```python
from build123d import *

# Parameters (mm, degrees)
ESBO_O1_R                = 45
RESSALTO_EXTRUS_O1_DEPTH = 50
ESBO_O2_R                = 4.5
CORTE_EXTRUS_O2_DEPTH    = 6
CORTE_EXTRUS_O3_DEPTH    = 7
ESBO_O4_W                = 40
ESBO_O4_H                = 15
CORTE_EXTRUS_O4_DEPTH    = 41
CORTE_EXTRUS_O5_START    = -6
ESBO_O5_R                = 4.5
CORTE_EXTRUS_O5_DEPTH    = 6
CORTE_EXTRUS_O6_START    = -7
CORTE_EXTRUS_O6_DEPTH    = 7
ESBO_O7_W                = 40
ESBO_O7_H                = 15
CORTE_EXTRUS_O7_DEPTH    = 47
CORTE_EXTRUS_O8_REACH    = 72.356
CORTE_EXTRUS_O9_REACH    = 72.356
ESBO_O9_W                = 5.8
ESBO_O9_H                = 3.2
ESBO_O11_W               = 40
ESBO_O11_H               = 15
ESBO_O11_W_2             = 13
ESBO_O11_H_2             = 7
RESSALTO_EXTRUS_O2_DEPTH = 22
ESBO_O12_R               = 1.6
CORTE_EXTRUS_O10_DEPTH   = 10
CORTE_EXTRUS_O11_REACH   = 75.614
ESBO_O13_R               = 4.5


with BuildPart() as part:
    # Esboço1 → Ressalto-extrusão1 (new body)
    with BuildSketch(Plane.XY):
        Circle(ESBO_O1_R)
    extrude(amount=RESSALTO_EXTRUS_O1_DEPTH)

    # Esboço2 → Corte-extrusão2 (cut)
    with BuildSketch(Plane.XY.offset(50)):
        Circle(ESBO_O2_R)
    extrude(amount=-CORTE_EXTRUS_O2_DEPTH, mode=Mode.SUBTRACT)

    # Esboço3 → Corte-extrusão3 (cut)
    with BuildSketch(Plane.XY.offset(44)):
        with BuildLine():
            Line((-6.5, -3.073450829), (-6.5, 7.19))
            Line((-6.5, 7.19), (6.5, 7.19))
            Line((6.5, 7.19), (6.5, -3.073450829))
            ThreePointArc((6.5, -3.073450829), (0, -7.19), (-6.5, -3.073450829))
        make_face()
    extrude(amount=-CORTE_EXTRUS_O3_DEPTH, mode=Mode.SUBTRACT)

    # Esboço4 → Corte-extrusão4 (cut)
    with BuildSketch(Plane.XZ.offset(-7.19)):
        with Locations((0, 37.5)):
            Rectangle(ESBO_O4_W, ESBO_O4_H)
    extrude(amount=-CORTE_EXTRUS_O4_DEPTH, mode=Mode.SUBTRACT)

    # Esboço5 → Corte-extrusão5 (cut)
    with BuildSketch(Plane(origin=(0, 0, 0), x_dir=(-1, 0, 0), z_dir=(0, 0, -1)).offset(CORTE_EXTRUS_O5_START)):
        with Locations(Location((0, 0, 0), (0, 0, 180))):
            Circle(ESBO_O5_R)
    extrude(amount=CORTE_EXTRUS_O5_DEPTH, mode=Mode.SUBTRACT)

    # Esboço6 → Corte-extrusão6 (cut)
    with BuildSketch(Plane(origin=(0, 0, 6), x_dir=(-1, 0, 0), z_dir=(0, 0, -1)).offset(CORTE_EXTRUS_O6_START)):
        with BuildLine():
            Line((-6.5, -3.073450829), (-6.5, 7.19))
            Line((-6.5, 7.19), (6.5, 7.19))
            Line((6.5, 7.19), (6.5, -3.073450829))
            ThreePointArc((6.5, -3.073450829), (0, -7.19), (-6.5, -3.073450829))
        make_face()
    extrude(amount=CORTE_EXTRUS_O6_DEPTH, mode=Mode.SUBTRACT)

    # Esboço7 → Corte-extrusão7 (cut)
    with BuildSketch(Plane.XZ.offset(-7.19)):
        with Locations((0, 12.5)):
            Rectangle(ESBO_O7_W, ESBO_O7_H)
    extrude(amount=-CORTE_EXTRUS_O7_DEPTH, mode=Mode.SUBTRACT)

    # Esboço8 → Corte-extrusão8 (cut, up to next)
    with BuildSketch(Plane.XY.offset(30), mode=Mode.PRIVATE) as corte_extrus_o8_sk1:
        Polygon((-20, 40.311288741), (-20, 47.3700993), (20, 47.3700993), (20, 40.311288741), (20, 37.311288741), (-20, 37.311288741), align=None)
    corte_extrus_o8_tool1 = extrude(corte_extrus_o8_sk1.sketch, amount=-CORTE_EXTRUS_O8_REACH, mode=Mode.PRIVATE) & part.part
    add(corte_extrus_o8_tool1.solids().sort_by_distance((0, 42.340694, 30))[0], mode=Mode.SUBTRACT)

    # Esboço9 → Corte-extrusão9 (cut, up to next)
    with BuildSketch(Plane(origin=(0, 0, 20), x_dir=(-1, 0, 0), z_dir=(0, 0, -1)), mode=Mode.PRIVATE) as corte_extrus_o9_sk1:
        with Locations((-15.1, 32.711288741)):
            Rectangle(ESBO_O9_W, ESBO_O9_H)
    corte_extrus_o9_tool1 = extrude(corte_extrus_o9_sk1.sketch, amount=-CORTE_EXTRUS_O9_REACH, mode=Mode.PRIVATE) & part.part
    # Esboço9 → Corte-extrusão9 (cut, up to next)
    with BuildSketch(Plane(origin=(0, 0, 20), x_dir=(-1, 0, 0), z_dir=(0, 0, -1)), mode=Mode.PRIVATE) as corte_extrus_o9_sk2:
        with Locations((15.1, 32.711288741)):
            Rectangle(ESBO_O9_W, ESBO_O9_H)
    corte_extrus_o9_tool2 = extrude(corte_extrus_o9_sk2.sketch, amount=-CORTE_EXTRUS_O9_REACH, mode=Mode.PRIVATE) & part.part
    add(corte_extrus_o9_tool1.solids().sort_by_distance((15.1, 32.711289, 20))[0], mode=Mode.SUBTRACT)
    add(corte_extrus_o9_tool2.solids().sort_by_distance((-15.1, 32.711289, 20))[0], mode=Mode.SUBTRACT)

    # Esboço11 → Ressalto-extrusão2 (add)
    # profile 1 of 2: a face of its own
    with BuildSketch(Plane(origin=(0, 7.19, 0), x_dir=(1, 0, 0), z_dir=(0, 1, 0))):
        with Locations((0, -12.5)):
            Rectangle(ESBO_O11_W, ESBO_O11_H)
        with Locations((0, -9.5)):
            Rectangle(ESBO_O11_W_2, ESBO_O11_H_2, mode=Mode.SUBTRACT)
    # profile 2 of 2: a face of its own
    with BuildSketch(Plane(origin=(0, 7.19, 0), x_dir=(1, 0, 0), z_dir=(0, 1, 0))):
        with Locations((0, -37.5)):
            Rectangle(ESBO_O11_W, ESBO_O11_H)
        with Locations((0, -40.5)):
            Rectangle(ESBO_O11_W_2, ESBO_O11_H_2, mode=Mode.SUBTRACT)
    extrude(amount=RESSALTO_EXTRUS_O2_DEPTH)

    # Esboço12 → Corte-extrusão10 (cut)
    with BuildSketch(Plane(origin=(0, 37.311288741, 0), x_dir=(1, 0, 0), z_dir=(0, 1, 0))):
        with Locations(Location((-15.1, -25, 0), (0, 0, 270))):
            Circle(ESBO_O12_R)
        with Locations(Location((15.1, -25, 0), (0, 0, 270))):
            Circle(ESBO_O12_R)
    extrude(amount=-CORTE_EXTRUS_O10_DEPTH, mode=Mode.SUBTRACT)

    # Esboço13 → Corte-extrusão11 (cut, up to next)
    with BuildSketch(Plane.XY.offset(37), mode=Mode.PRIVATE) as corte_extrus_o11_sk1:
        Circle(ESBO_O13_R)
    corte_extrus_o11_tool1 = extrude(corte_extrus_o11_sk1.sketch, amount=-CORTE_EXTRUS_O11_REACH, mode=Mode.PRIVATE) & part.part
    add(corte_extrus_o11_tool1.solids().sort_by_distance((0, 0, 37))[0], mode=Mode.SUBTRACT)


solid = part.part
```
Geometry: final body of the model. Coordinates: model frame, mm. A direction names the side the tool comes from. Give positions to 0.01 mm unless a question says otherwise; leave off trailing zeros. Loops run counter-clockwise (first coordinate to the right, second up) from the corner with the lowest first, then second, coordinate; pieces in that order, holes last. Notation, with made-up numbers: (-2.5, 33.5) -> (1.5, 33.5) arc R14 cw to (1.5, 45.5) -> close; hole circle Ø6 at (61, 74.5). An arc over 180 degrees is marked (long way). Use CSV: the item, a comma, the result in double quotes.
(1) Pull-direction query (Y, two-part tool) for faces 4 (the face through (18, 33, 25)), 5 (the face through (0, 33, 20)), 6 (the face through (20.765, -39.923, 24.65)); classes: released by +Y, released by -Y, zero draft, split by the parting line, or undercut.
From the geometry:
face 4,"undercut"
face 5,"zero draft"
face 6,"split by the parting line"
(2) Cut plane C-C (z = 39). Output: boundary loops of the cut face in (x, y).
From the geometry:
outline,"(-20, 29.19) -> (-20, 40.31) arc R45 ccw (long way) to (20, 40.31) -> (20, 29.19) -> (6.5, 29.19) -> (6.5, -3.07) arc R7.19 cw to (-6.5, -3.07) -> (-6.5, 29.19) -> close"
(3) First-contact query: P1, Ø6.5, axis at x = -14, z = 22.5, coming from the +Y side; P2, Ø12, axis at y = -14, z = 30.5, coming from the +X side; P3, Ø8, axis at x = -22.5, z = 11.5, coming from the -Y side; P4, Ø7, axis at x = 0, y = 0, coming from the +Z side. Flat tips, straight axial feed; report the tip coordinate or a pass-through.
From the geometry:
P1,"y = 37.31"
P2,"x = 44.28"
P3,"y = -41.02"
P4,"through"
(4) Access query for faces 1 (the face through (-0.11, -7.19, 9.55)), 2 (the face through (-18, 33, 25)), 3 (the face through (-3.32, -3.04, 3.04)). Directions: +Z, -Z, +X, -X, +Y, -Y. A direction counts if a zero-diameter tool reaches every point of the face in a straight line with its end or side. Return the directions, or none.
From the geometry:
face 1,"+Y"
face 2,"none"
face 3,"+Z, -Z"
(5) Cut plane B-B (y = 0). Output: boundary loops of the cut face in (x, z), plus the area to 3 significant figures.
From the geometry:
outline,"(-45, 0) -> (-4.5, 0) -> (-4.5, 6) -> (-6.5, 6) -> (-6.5, 13) -> (-4.5, 13) -> (-4.5, 37) -> (-6.5, 37) -> (-6.5, 44) -> (-4.5, 44) -> (-4.5, 50) -> (-45, 50) -> close; (4.5, 0) -> (45, 0) -> (45, 50) -> (4.5, 50) -> (4.5, 44) -> (6.5, 44) -> (6.5, 37) -> (4.5, 37) -> (4.5, 13) -> (6.5, 13) -> (6.5, 6) -> (4.5, 6) -> close"
area,"3,990 mm^2"
(6) Cut plane D-D (y = 10). Output: boundary loops of the cut face in (x, z).
From the geometry:
outline,"(-43.87, 0) -> (43.87, 0) -> (43.87, 50) -> (-43.87, 50) -> close; hole (-6.5, 6) -> (6.5, 6) -> (6.5, 13) -> (-6.5, 13) -> close; hole (-6.5, 37) -> (6.5, 37) -> (6.5, 44) -> (-6.5, 44) -> close"
(7) Ray query, line 1 along Z through (x, y) = (15, 35); line 2 along Y through (x, z) = (0, 48.7); line 3 along Z through (x, y) = (1, 14). Return the intervals inside material, ascending. Write a range as [from, to].
From the geometry:
line 1,"[0, 5], [20, 23.4], [26.6, 30], [45, 50]"
line 2,"[-45, -4.5], [4.5, 45]"
line 3,"[0, 6], [13, 37], [44, 50]"
(8) Cut plane A-A (x = 0). Count the separate pieces of the cut face and the enclosed holes in it, plus the area to 3 significant figures.
From the geometry:
separate pieces,"4"
enclosed holes,"0"
area,"3,120 mm^2"
